from build123d import *

# Parameters (mm, degrees)
SKETCH1_R           = 1.55
BOSS_EXTRUDE1_DEPTH = 10
SKETCH3_W           = 15.2
SKETCH3_H           = 132
CUT_EXTRUDE1_DEPTH  = 5
SKETCH4_W           = 9.7
SKETCH4_H           = 93
CUT_EXTRUDE2_DEPTH  = 2
CUT_EXTRUDE4_DEPTH  = 2.3


with BuildPart() as part:
    # Sketch1 → Boss-Extrude1 (new body)
    with BuildSketch(Plane(origin=(0, 0, 0), x_dir=(1, 0, 0), z_dir=(0, 1, 0))):
        Polygon((0, 0), (7.3, 0), (7.3, 17), (22.5, 17), (22.5, 36.5), (17, 36.5), (17, 57), (7.3, 57), (7.3, 109), (17, 109), (17, 129.5), (22.5, 129.5), (22.5, 149), (7.3, 149), (7.3, 166), (0, 166), (0, 163), (4, 163), (4, 3), (0, 3), align=None)
        with Locations((17, 25.85)):
            Circle(SKETCH1_R, mode=Mode.SUBTRACT)
        with Locations((12, 44.9)):
            Circle(SKETCH1_R, mode=Mode.SUBTRACT)
        with Locations((12, 121.1)):
            Circle(SKETCH1_R, mode=Mode.SUBTRACT)
        with Locations((17, 140.15)):
            Circle(SKETCH1_R, mode=Mode.SUBTRACT)
    extrude(amount=BOSS_EXTRUDE1_DEPTH)

    # Sketch3 → Cut-Extrude1 (cut)
    with BuildSketch(Plane(origin=(0, 10, 0), x_dir=(1, 0, 0), z_dir=(0, 1, 0))):
        with Locations((14.9, 83)):
            Rectangle(SKETCH3_W, SKETCH3_H)
    extrude(amount=-CUT_EXTRUDE1_DEPTH, mode=Mode.SUBTRACT)

    # Sketch4 → Cut-Extrude2 (cut)
    with BuildSketch(Plane(origin=(0, 5, 0), x_dir=(1, 0, 0), z_dir=(0, 1, 0))):
        with Locations((12.15, 83)):
            Rectangle(SKETCH4_W, SKETCH4_H)
    extrude(amount=-CUT_EXTRUDE2_DEPTH, mode=Mode.SUBTRACT)

    # Sketch5 → Cut-Extrude4 (cut)
    with BuildSketch(Plane.XZ):
        Polygon((19.75, -24.26228676), (19.75, -27.43771324), (17, -29.025426481), (14.25, -27.43771324), (14.25, -24.26228676), (17, -22.674573519), align=None)
        Polygon((14.25, -138.56228676), (14.25, -141.73771324), (17, -143.325426481), (19.75, -141.73771324), (19.75, -138.56228676), (17, -136.974573519), align=None)
    extrude(amount=-CUT_EXTRUDE4_DEPTH, mode=Mode.SUBTRACT)


solid = part.part
Check sheet for the modelled part. Datum: model origin and axes. Units: mm. A direction names the side the tool comes from. Give positions to 0.01 mm unless a question says otherwise; leave off trailing zeros. Order: outer loops, then holes, each group sorted by start corner. A loop starts at its lowest first (then second) coordinate and runs counter-clockwise, first axis right, second up. Notation, with made-up numbers: M 82.5,-26.5 L 134.5,-26.5 A14 cw 134.5,-0.5 Z; hole C -13,-30 d9. An arc over 180 degrees is marked long. Answer as CSV lines item,"result". Start each with the question number.
Item 1: Cross-section at D-D on x = 12. Enter the section's corners in (y, z).
Item 2: Tool access check on faces 1 (the face through (17, 1, -47)), 2 (the face through (16, 2.3, -24)), 3 (the face through (12, 3, -119)). Record the directions out of +Z, -Z, +X, -X, +Y, -Y that give a thin tool (end or side, any length) a straight path to the whole face; none if there is none.
Item 3: Cross-section at A-A on z = -44.9. Enter the section's corners in (x, y), plus the area to 3 significant figures.
Item 4: Mould release check, pull along X, two halves, no side actions. Record for faces 4 (the face through (4, 5, -84)), 5 (the face through (5, 0, -83)), 6 (the face through (18, 2.3, -142)): +X half, -X half, draft (parallel to the pull), parting line (faces both ways), or undercut.
Item 5: Gauge pin test, flat ends, axial feed: P1, Ø3, axis at y = 2, z = -115.5, coming from the +X side; P2, Ø0.7, axis at y = 1.5, z = -25.5, coming from the -X side; P3, Ø3.5, axis at x = 13.5, y = 1.5, coming from the -Z side. Record the tip position at first contact, or that the pin passes through.
Item 6: Thickness scan on line 1 (Z direction, x = 12, y = 0.8); line 2 (Z direction, x = 17, y = 4.4); line 3 (X direction, y = 1.4, z = -44.9). Record the ranges inside material, lowest first. Write a range as [from, to].
Item 7: Cross-section at C-C on y = 8. Enter the section's corners in (x, z).
Item 8: Cross-section at B-B on x = 2. Enter the section's corners in (y, z), plus the area to 3 significant figures.
Established:
1,outline,"M 0,-149 L 5,-149 L 5,-129.5 L 3,-129.5 L 3,-122.65 L 0,-122.65 Z; M 0,-119.55 L 3,-119.55 L 3,-109 L 0,-109 Z; M 0,-57 L 3,-57 L 3,-46.45 L 0,-46.45 Z; M 0,-43.35 L 3,-43.35 L 3,-36.5 L 5,-36.5 L 5,-17 L 0,-17 Z"
2,face 1,"+X, +Y, -Y"
2,face 2,"-Y"
2,face 3,"+X, +Y"
3,outline,"M 4,0 L 10.45,0 L 10.45,3 L 7.3,3 L 7.3,10 L 4,10 Z; M 13.55,0 L 17,0 L 17,3 L 13.55,3 Z"
3,area,"52.8 mm^2"
4,face 4,"-X half"
4,face 5,"draft"
4,face 6,"undercut"
5,P1,"stops at x = 17"
5,P2,"stops at x = 4"
5,P3,"stops at z = -149"
6,line 1,"z = [-149, -122.65], [-119.55, -109], [-57, -46.45], [-43.35, -17]"
6,line 2,"z = [-149, -141.7], [-138.6, -129.5], [-36.5, -27.4], [-24.3, -17]"
6,line 3,"x = [4, 10.45], [13.55, 17]"
7,outline,"M 0,-166 L 7.3,-166 L 7.3,0 L 0,0 L 0,-3 L 4,-3 L 4,-163 L 0,-163 Z"
8,outline,"M 0,-166 L 10,-166 L 10,-163 L 0,-163 Z; M 0,-3 L 10,-3 L 10,0 L 0,0 Z"
8,area,"60.0 mm^2"
